```python
from build123d import *

# Parameters (mm, degrees)
F1_DEPTH = 483.87
F2_R     = 127
F3_R     = 127
F5_DEPTH = 262.8959715366
F6_R     = 38.1
F7_DEPTH = 111.5219220519


with BuildPart() as f1:
    # F0 (on Front) → F1 (new body)
    with BuildSketch(Plane.XZ):
        with BuildLine():
            Line((1270, -41.7147416453), (79.7203516274, -41.7147416453))
            ThreePointArc((79.7203516274, -41.7147416453), (46.5949623447, -76.9698877369), (0, -89.9747416453))
            Line((0, -89.9747416453), (1270, -89.9747416453))
            Line((1270, -89.9747416453), (1270, -41.7147416453))
        make_face()
        with BuildLine():
            ThreePointArc((-63.6217499529, 63.6217499529), (-21.4783157229, 87.373543409), (26.8740245415, 85.8675779271))
            Line((26.8740245415, 85.8675779271), (92.6755573214, 151.669110707))
            Line((92.6755573214, 151.669110707), (419.5160293606, 478.5095827463))
            Line((419.5160293606, 478.5095827463), (385.3910561006, 512.6345560063))
            Line((385.3910561006, 512.6345560063), (-63.6217499529, 63.6217499529))
        make_face()
        with BuildLine():
            ThreePointArc((0, -41.7147416453), (-38.5393960101, -15.963540513), (-29.4967766928, 29.4967766928))
            Line((-29.4967766928, 29.4967766928), (26.8740245415, 85.8675779271))
            ThreePointArc((26.8740245415, 85.8675779271), (-21.4783157229, 87.373543409), (-63.6217499529, 63.6217499529))
            ThreePointArc((-63.6217499529, 63.6217499529), (-83.1258222491, -34.431842959), (0, -89.9747416453))
            ThreePointArc((0, -89.9747416453), (46.5949623447, -76.9698877369), (79.7203516274, -41.7147416453))
            Line((79.7203516274, -41.7147416453), (0, -41.7147416453))
        make_face()
    extrude(amount=F1_DEPTH)

    # F2
    f2_edges = [f1.edges().sort_by_distance(p)[0] for p in [
        (1270, -483.87, -65.844742),
        (1270, 0, -65.844742),
    ]]
    fillet(f2_edges, radius=F2_R)

    # F3
    f3_edges = [f1.edges().sort_by_distance(p)[0] for p in [
        (402.453543, -483.87, 495.572069),
        (402.453543, 0, 495.572069),
    ]]
    fillet(f3_edges, radius=F3_R)

    # F4 (on Top) → F5 (cut)
    with BuildSketch(Plane.XY):
        with BuildLine():
            ThreePointArc((768.1907979278, -178.435), (766.9421834827, -178.4227264611), (765.6935690377, -178.435))
            Line((765.6935690377, -178.435), (768.1907979278, -178.435))
        make_face()
        with BuildLine():
            Line((768.1907979278, -178.435), (765.6935690377, -178.435))
            ThreePointArc((765.6935690377, -178.435), (721.5907686724, -197.4682971963), (703.4238827535, -241.935))
            Line((703.4238827535, -241.935), (703.4238827535, -241.9470549528))
            ThreePointArc((703.4238827535, -241.9470549528), (721.412813036, -286.2315568319), (765.1843390533, -305.435))
            Line((765.1843390533, -305.435), (768.7000279122, -305.435))
            Line((768.7000279122, -305.435), (1087.7811908722, -305.435))
            Line((1087.7811908722, -305.435), (1114.4740463012, -305.435))
            ThreePointArc((1114.4740463012, -305.435), (1150.8110443569, -283.3041158357), (1165.3364646129, -243.3145468461))
            Line((1165.3364646129, -243.3145468461), (1165.3364646129, -241.935))
            ThreePointArc((1165.3364646129, -241.935), (1146.8921429081, -197.581904853), (1102.8377891298, -178.435))
            Line((1102.8377891298, -178.435), (1099.4174480436, -178.435))
            Line((1099.4174480436, -178.435), (768.1907979278, -178.435))
        make_face()
        with BuildLine():
            ThreePointArc((1102.8377891298, -178.435), (1101.1276185867, -178.4122225051), (1099.4174480436, -178.435))
            Line((1099.4174480436, -178.435), (1102.8377891298, -178.435))
        make_face()
        with BuildLine():
            Line((768.7000279122, -305.435), (765.1843390533, -305.435))
            ThreePointArc((765.1843390533, -305.435), (766.9421834827, -305.4593284917), (768.7000279122, -305.435))
        make_face()
        with BuildLine():
            ThreePointArc((1165.3364646129, -243.3145468461), (1165.3401695046, -242.624773423), (1165.3364646129, -241.935))
            Line((1165.3364646129, -241.935), (1165.3364646129, -243.3145468461))
        make_face()
        with BuildLine():
            Line((1114.4740463012, -305.435), (1087.7811908722, -305.435))
            ThreePointArc((1087.7811908722, -305.435), (1101.1276185867, -306.837324341), (1114.4740463012, -305.435))
        make_face()
        with BuildLine():
            ThreePointArc((460.0986740112, -175.5972226858), (415.1973934059, -283.9985032912), (523.5986740112, -239.0972226858))
            ThreePointArc((523.5986740112, -239.0972226858), (504.9999546166, -194.1959420805), (460.0986740112, -175.5972226858))
        make_face()
    extrude(amount=-F5_DEPTH, mode=Mode.SUBTRACT)

    # F6 (on face) → F7 (cut)
    with BuildSketch(Plane(origin=(-63.6217499529, 0, 63.6217499529), x_dir=(0, -1, 0), z_dir=(-0.7071067812, 0, 0.7071067812))):
        with Locations((114.3, 457.2814617571)):
            Circle(F6_R)
        with Locations((369.57, 457.2)):
            Circle(F6_R)
    extrude(amount=-F7_DEPTH, mode=Mode.SUBTRACT)


solid = f1.part
```
Model file for the job. Use its own axes, mm. A direction names the side the tool comes from. Give positions to 0.01 mm unless a question says otherwise; leave off trailing zeros. Order: outer loops, then holes, each group sorted by start corner. A loop starts at its lowest first (then second) coordinate and runs counter-clockwise, first axis right, second up.
1) Mould opens along X. For faces 6 (the flat face through (926, -305.435, -66)), 7 (the flat face through (191.867, -238.548, 250.86)), 8 (the cylindrical face through (-83.68, -238.55, -33.06)) say: +X half, -X half, draft (parallel to the pull), parting line (faces both ways), or undercut.
2) Pin check, flat tips, straight feed: pin 1 (8 mm diameter, centred on y = -357, z = 432, fed in from +X); pin 2 (12 mm diameter, centred on x = 976, y = -342, fed in from +Z); pin 3 (4 mm diameter, centred on y = -230.5, z = 41, fed in from +X). Stop position of each tip, or through.
3) Saw through at C-C, the plane y = -431.5. Write the cut outline in (x, z).
4) Saw through at B-B, the plane y = -279. Write the cut outline in (x, z), then the cut area to 3 significant figures.
5) Saw through at A-A, the plane x = 830. Write the cut outline in (y, z) (3 decimals), then the cut area to 3 significant figures.
6) Saw through at D-D, the plane x = 446. Write the cut outline in (y, z), then the cut area to 3 significant figures.
7) 3-axis set-ups, long thin cutter, end or side, ignore diameter. For faces 1 (the flat face through (936, -178.435, -66)), 2 (the cylindrical face through (520.666, -220.024, -65.507)), 3 (the flat face through (341, -483.87, -60)), 4 (the flat face through (644, -239, -41.715)), 5 (the flat face through (626, -239, -89.975)): which of +Z, -Z, +X, -X, +Y, -Y reach the whole face in a straight line?
8) Wall check: probe 1 along Z at (x, y) = (502, -172); probe 2 along X at (y, z) = (-325.5, -5); probe 3 along Z at (x, y) = (375, -296). Give the ranges that are in metal, low to high.
Computed:
1. face 6: undercut
1. face 7: +X half
1. face 8: -X half
2. pin 1: stops at x = 377.01
2. pin 2: stops at z = -41.71
2. pin 3: stops at x = -15.99
3. outline: (-63.62, 63.62) arc R89.97 ccw to (0, -89.97) - (1245.76, -89.97) - (1245.76, -41.71) - (0, -41.71) arc R41.71 cw to (-29.5, 29.5) - (402.37, 461.37) - (368.25, 495.49) - close
4. outline: (-63.62, 63.62) arc R89.97 ccw to (0, -89.97) - (410.7, -89.97) - (410.7, -41.71) - (0, -41.71) arc R41.71 cw to (-29.5, 29.5) - (419.52, 478.51) - (385.39, 512.63) - close; (509.5, -89.97) - (715.36, -89.97) - (715.36, -41.71) - (509.5, -41.71) - close; (1154.04, -89.97) - (1270, -89.97) - (1270, -41.71) - (1154.04, -41.71) - close
4. area: 73,500 mm2
5. outline: (-483.87, -89.975) - (-305.435, -89.975) - (-305.435, -41.715) - (-483.87, -41.715) - close; (-178.435, -89.975) - (0, -89.975) - (0, -41.715) - (-178.435, -41.715) - close
5. area: 17,200 mm2
6. outline: (-483.87, -89.97) - (-301.01, -89.97) - (-301.01, -41.71) - (-483.87, -41.71) - close; (-177.18, -89.97) - (0, -89.97) - (0, -41.71) - (-177.18, -41.71) - close
6. area: 17,400 mm2
7. face 1: +Z, -Z
7. face 2: -Z
7. face 3: +Z, -Z, +X, -X, -Y
7. face 4: +X, +Y, -Y
7. face 5: -Z, +X, -X, +Y, -Y
8. probe 1: z = -89.97 to -41.71
8. probe 2: x = -89.84 to -41.41
8. probe 3: z = -89.97 to -41.71, 433.99 to 502.24
